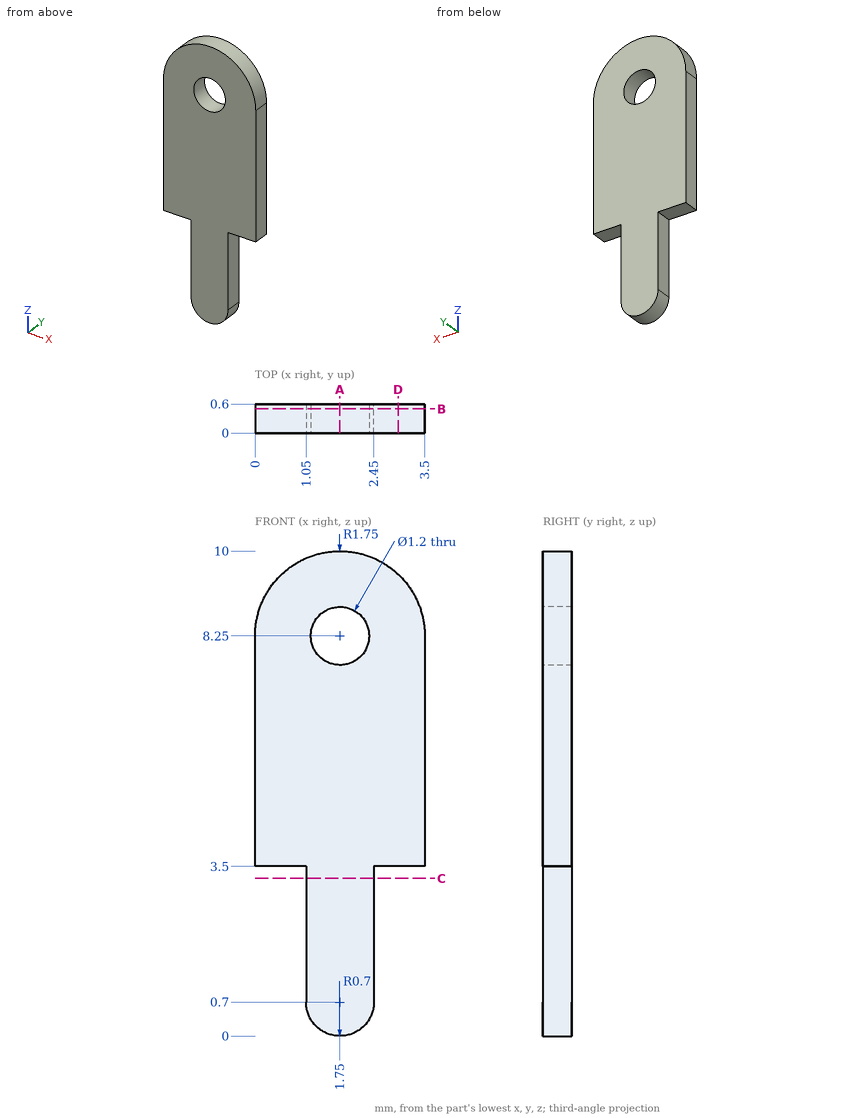
Verification items for this drawing (mm, ordinates from the low corner). Give positions to 0.01 mm unless a question says otherwise; leave off trailing zeros. Loops run counter-clockwise (first coordinate to the right, second up) from the corner with the lowest first, then second, coordinate; pieces in that order, holes last. Notation, with made-up numbers: M 37.25,42.5 L 55.25,42.5 A23 cw 55.25,66.5 Z; hole C 20.5,28.25 d10. An arc over 180 degrees is marked long. Answer in a Markdown table with one row per item.
1) Cross-section at A-A (x = 1.75). Enter the section's corners in (y, z).
Solutions:
| item | result |
|---|---|
| outline | M 0,0 L 0.6,0 L 0.6,7.65 L 0,7.65 Z; M 0,8.85 L 0.6,8.85 L 0.6,10 L 0,10 Z |
2) Cross-section at B-B (y = 0.5). Enter the section's corners in (x, z), plus the area to 3 significant figures.
Solutions:
| item | result |
|---|---|
| outline | M 0,3.5 L 1.05,3.5 L 1.05,0.7 A0.7 ccw 2.45,0.7 L 2.45,3.5 L 3.5,3.5 L 3.5,8.25 A1.75 ccw 0,8.25 Z; hole C 1.75,8.25 d1.2 |
| area | 25.0 mm^2 |
3) Thickness scan on line 1 (Z direction, x = 1.75, y = 0.25); line 2 (X direction, y = 0.4, z = 1); line 3 (X direction, y = 0.4, z = 8.75). Record the ranges inside material, lowest first.
Solutions:
| item | result |
|---|---|
| line 1 | z = 0 to 7.65, 8.85 to 10 |
| line 2 | x = 1.05 to 2.45 |
| line 3 | x = 0.07 to 1.42, 2.08 to 3.43 |
4) Cross-section at C-C (z = 3.25). Enter the section's corners in (x, y), plus the area to 3 significant figures.
Solutions:
| item | result |
|---|---|
| outline | M 1.05,0 L 2.45,0 L 2.45,0.6 L 1.05,0.6 Z |
| area | 0.840 mm^2 |
5) Cross-section at D-D (x = 2.95). Enter the section's corners in (y, z), plus the area to 3 significant figures.
Solutions:
| item | result |
|---|---|
| outline | M 0,3.5 L 0.6,3.5 L 0.6,9.52 L 0,9.52 Z |
| area | 3.61 mm^2 |
